from build123d import *

# Parameters (mm, degrees)
EXTRUDE_THIN1_DEPTH = 17.5
BOSS_EXTRUDE2_DEPTH = 7
BOSS_EXTRUDE3_START = -59
BOSS_EXTRUDE3_DEPTH = 7
FILLET1_R           = 3
CUT_EXTRUDE1_START  = -7
CUT_EXTRUDE1_DEPTH  = 2
CUT_EXTRUDE2_START  = -66
CUT_EXTRUDE2_DEPTH  = 7
CUT_EXTRUDE3_REACH  = 87.636
SKETCH4_R           = 2.5
CUT_EXTRUDE4_REACH  = 87.636
SKETCH4_3_R         = 1.5
CIRPATTERN1_COUNT   = 4


with BuildPart() as part:
    # Sketch2 → Extrude-Thin1 (new, symmetric)
    with BuildSketch(Plane.XY):
        Polygon((-33, 40), (-33, 0), (33, 0), (33, 40), (26, 40), (26, 7), (-26, 7), (-26, 40), align=None)
    extrude(amount=EXTRUDE_THIN1_DEPTH, both=True)

    # Sketch3 → Boss-Extrude2 (add)
    with BuildSketch(Plane.ZY.offset(33)):
        with BuildLine():
            Line((11.25, 40), (17.5, 40))
            ThreePointArc((17.5, 40), (0, 57.5), (-17.5, 40))
            Line((-17.5, 40), (-11.25, 40))
            ThreePointArc((-11.25, 40), (0, 51.25), (11.25, 40))
        make_face()
        with BuildLine():
            ThreePointArc((-17.5, 40), (0, 22.5), (17.5, 40))
            Line((17.5, 40), (11.25, 40))
            ThreePointArc((11.25, 40), (0, 28.75), (-11.25, 40))
            Line((-11.25, 40), (-17.5, 40))
        make_face()
        with BuildLine():
            Line((-11.25, 40), (11.25, 40))
            ThreePointArc((11.25, 40), (0, 51.25), (-11.25, 40))
        make_face()
        with BuildLine():
            ThreePointArc((-11.25, 40), (0, 28.75), (11.25, 40))
            Line((11.25, 40), (-11.25, 40))
        make_face()
    extrude(amount=-BOSS_EXTRUDE2_DEPTH)

    # Sketch3<3> → Boss-Extrude3 (add)
    with BuildSketch(Plane.ZY.offset(33).offset(BOSS_EXTRUDE3_START)):
        with BuildLine():
            Line((-11.25, 40), (11.25, 40))
            ThreePointArc((11.25, 40), (0, 51.25), (-11.25, 40))
        make_face()
        with BuildLine():
            ThreePointArc((-11.25, 40), (0, 28.75), (11.25, 40))
            Line((11.25, 40), (-11.25, 40))
        make_face()
        with BuildLine():
            Line((11.25, 40), (17.5, 40))
            ThreePointArc((17.5, 40), (0, 57.5), (-17.5, 40))
            Line((-17.5, 40), (-11.25, 40))
            ThreePointArc((-11.25, 40), (0, 51.25), (11.25, 40))
        make_face()
        with BuildLine():
            ThreePointArc((-17.5, 40), (0, 22.5), (17.5, 40))
            Line((17.5, 40), (11.25, 40))
            ThreePointArc((11.25, 40), (0, 28.75), (-11.25, 40))
            Line((-11.25, 40), (-17.5, 40))
        make_face()
    extrude(amount=-BOSS_EXTRUDE3_DEPTH)

    # Fillet1
    fillet1_edges = [part.edges().sort_by_distance(p)[0] for p in [
        (-26, 7, 0),
        (26, 7, 0),
        (33, 0, 0),
        (-33, 0, 0),
        (-33, 20, 17.5),
        (0, 0, 17.5),
        (33, 20, 17.5),
        (-33, 57.5, 0),
        (-26, 57.5, 0),
        (26, 23.5, 17.5),
        (33, 57.5, 0),
        (26, 57.5, 0),
        (0, 7, 17.5),
        (-26, 23.5, 17.5),
        (0, 7, -17.5),
        (26, 23.5, -17.5),
        (33, 20, -17.5),
        (0, 0, -17.5),
        (-33, 20, -17.5),
        (-26, 23.5, -17.5),
    ]]
    fillet(fillet1_edges, radius=FILLET1_R)

    # Sketch3<4> → Cut-Extrude1 (cut)
    with BuildSketch(Plane.ZY.offset(33).offset(CUT_EXTRUDE1_START)):
        with BuildLine():
            Line((-11.25, 40), (11.25, 40))
            ThreePointArc((11.25, 40), (0, 51.25), (-11.25, 40))
        make_face()
        with BuildLine():
            ThreePointArc((-11.25, 40), (0, 28.75), (11.25, 40))
            Line((11.25, 40), (-11.25, 40))
        make_face()
    extrude(amount=CUT_EXTRUDE1_DEPTH, mode=Mode.SUBTRACT)

    # Sketch3<5> → Cut-Extrude2 (cut)
    with BuildSketch(Plane.ZY.offset(33).offset(CUT_EXTRUDE2_START)):
        with BuildLine():
            Line((-11.25, 40), (11.25, 40))
            ThreePointArc((11.25, 40), (0, 51.25), (-11.25, 40))
        make_face()
        with BuildLine():
            ThreePointArc((-11.25, 40), (0, 28.75), (11.25, 40))
            Line((11.25, 40), (-11.25, 40))
        make_face()
    extrude(amount=CUT_EXTRUDE2_DEPTH, mode=Mode.SUBTRACT)

    # Sketch4 → Cut-Extrude3 (cut, up to next)
    with BuildSketch(Plane(origin=(-28, 0, 0), x_dir=(0, 0, -1), z_dir=(1, 0, 0)), mode=Mode.PRIVATE) as cut_extrude3_sk1:
        with Locations(Location((0, 40, 0), (0, 0, 90))):
            Circle(SKETCH4_R)
    cut_extrude3_tool1 = extrude(cut_extrude3_sk1.sketch, amount=-CUT_EXTRUDE3_REACH, mode=Mode.PRIVATE) & part.part
    add(cut_extrude3_tool1.solids().sort_by_distance((-28, 40, 0))[0], mode=Mode.SUBTRACT)

    # Sketch4<3> → Cut-Extrude4 (cut, up to next)
    with BuildSketch(Plane(origin=(-28, 0, 0), x_dir=(0, 0, -1), z_dir=(1, 0, 0)), mode=Mode.PRIVATE) as cut_extrude4_sk1:
        with Locations(Location((7, 40, 0), (0, 0, 90))):
            Circle(SKETCH4_3_R)
    cut_extrude4_tool1 = extrude(cut_extrude4_sk1.sketch, amount=-CUT_EXTRUDE4_REACH, mode=Mode.PRIVATE) & part.part
    cut_extrude4 = cut_extrude4_tool1.solids().sort_by_distance((-28, 40, -7))[0]
    add(cut_extrude4, mode=Mode.SUBTRACT)

    # CirPattern1: Cut-Extrude4 ×4 about axis
    cirpattern1_axis = Axis((0, 40, 0), (1, 0, 0))
    for i in range(1, CIRPATTERN1_COUNT):
        add(cut_extrude4.rotate(cirpattern1_axis, i * 360 / CIRPATTERN1_COUNT), mode=Mode.SUBTRACT)


solid = part.part
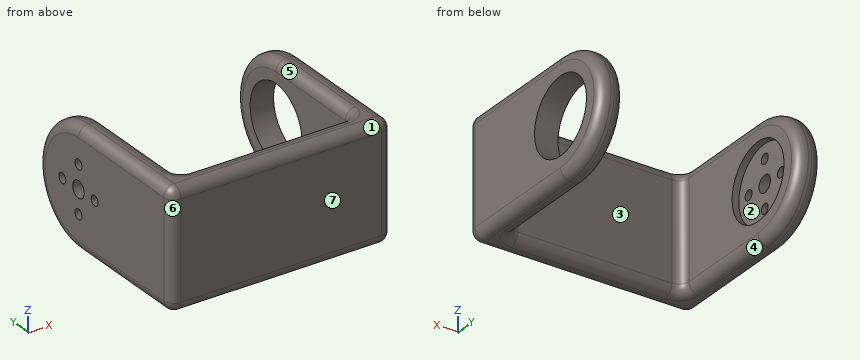
Could you check a few things on this model? Use its own coordinates, in mm. Face numbers are marked on the shaded views. A direction names the side the tool comes from. Give positions to 0.01 mm unless a question says otherwise; leave off trailing zeros. Order: outer loops, then holes, each group sorted by start corner. A loop starts at its lowest first (then second) coordinate and runs counter-clockwise, first axis right, second up. Notation, with made-up numbers: (55.25, -40) -> (78.25, -40) arc R20 cw to (78.25, -20) -> close; hole circle Ø3 at (79, -27). An arc over 180 degrees is marked (long way). Return JSON: item names as keys, results as strings.
1. For pin 1 Ø1.5 at (x, z) = (-8, 13) entering from +Y; pin 2 Ø20 at (y, z) = (40, 0) entering from +X, each with a flat end and sliding along its axis, tell me the tip position at first contact or that it passes through.
Answer list:
{"pin 1": "stops at y = 7", "pin 2": "stops at x = -28"}
2. Imagine slicing it at A-A on y = 19.5. List the corners of the cut face in (x, z) for me.
Answer list:
{"outline": "(-33, -14.5) arc R3 ccw to (-30, -17.5) -> (-29, -17.5) arc R3 ccw to (-26, -14.5) -> (-26, 14.5) arc R3 ccw to (-29, 17.5) -> (-30, 17.5) arc R3 ccw to (-33, 14.5) -> close; (26, -14.5) arc R3 ccw to (29, -17.5) -> (30, -17.5) arc R3 ccw to (33, -14.5) -> (33, 14.5) arc R3 ccw to (30, 17.5) -> (29, 17.5) arc R3 ccw to (26, 14.5) -> close"}
3. Thinking about a two-plate mould opening in X: for the marked faces 5, 6 and 7, which applies, pulls with the +X half, pulls with the -X half, needs draft (parallel to the pull), parting line crosses it, or undercut?
Answer list:
{"face 5": "undercut", "face 6": "pulls with the -X half", "face 7": "needs draft"}
4. I need wall thicknesses on line 1 (X direction, y = 16, z = -13); line 2 (Z direction, x = -31.3, y = 40); line 3 (X direction, y = 38, z = 11). Which ranges of each line are inside material? Lowest first, please. Write a range as from..to.
Answer list:
{"line 1": "x = -33..-26, 26..33", "line 2": "z = -17.2..-8.5, -5.5..-2.5, 2.5..5.5, 8.5..17.2", "line 3": "x = -33..-28"}
5. Imagine slicing it at D-D on z = 0. Give the number of separate pieces and of enclosed holes in the cut face, then the cut area to 3 significant figures.
Answer list:
{"separate pieces": "5", "enclosed holes": "0", "area": "904 mm2"}
6. Imagine slicing it at B-B on x = -21.5. List the corners of the cut face in (y, z) for me.
Answer list:
{"outline": "(0, -14.5) arc R3 ccw to (3, -17.5) -> (4, -17.5) arc R3 ccw to (7, -14.5) -> (7, 14.5) arc R3 ccw to (4, 17.5) -> (3, 17.5) arc R3 ccw to (0, 14.5) -> close"}
7. On a 3-axis mill with a long thin cutter (end or side, diameter ignored), from which of +Z, -Z, +X, -X, +Y, -Y can I reach the whole of each face in a straight line? I mean the marked faces 1, 2, 3 and 4. Say none if no direction works.
Answer list:
{"face 1": "+Z, +X, -X, -Y", "face 2": "+X", "face 3": "+Z, -Z, +Y", "face 4": "-Z, +Y"}
8. Imagine slicing it at C-C on y = 33. List the corners of the cut face in (x, z) for me, then the cut area to 3 significant figures.
Answer list:
{"outline": "(-33, -14.5) arc R3 ccw to (-30, -17.5) -> (-29, -17.5) arc R3 ccw to (-26, -14.5) -> (-26, -8.81) -> (-28, -8.81) -> (-28, -1.5) -> (-33, -1.5) -> close; (-33, 1.5) -> (-28, 1.5) -> (-28, 8.81) -> (-26, 8.81) -> (-26, 14.5) arc R3 ccw to (-29, 17.5) -> (-30, 17.5) arc R3 ccw to (-33, 14.5) -> close; (26, -14.5) arc R3 ccw to (29, -17.5) -> (30, -17.5) arc R3 ccw to (33, -14.5) -> (33, -8.81) -> (26, -8.81) -> close; (26, 8.81) -> (33, 8.81) -> (33, 14.5) arc R3 ccw to (30, 17.5) -> (29, 17.5) arc R3 ccw to (26, 14.5) -> close", "area": "301 mm2"}
